Verification items for the finished model (mm, model axes). Face numbers are marked on the shaded views. A direction names the side the tool comes from. Round coordinates to 2 decimals unless told otherwise and drop trailing zeros. Order: outer loops, then holes, each group sorted by start corner. A loop starts at its lowest first (then second) coordinate and runs counter-clockwise, first axis right, second up. Notation, with made-up numbers: M 39.25,13.25 L 71.25,13.25 A23 cw 71.25,37.25 Z; hole C -13.5,-25 d3. An arc over 180 degrees is marked long. Use CSV: the item, a comma, the result in double quotes. Start each with the question number.
Q1. Sectioned sample at C-C (x = 8.25). Enter the section's corners in (y, z).
Q2. Gauge pin test, flat end, axial feed: pin 1 Ø3 at (x, z) = (2, 6.5) entering from -Y. Record the tip position at first contact, or that the pin passes through.
Q3. Set-up check for the marked faces 1 and 2: record each of +Z, -Z, +X, -X, +Y, -Y from which the full face is reachable in a straight line by a thin tool's end or side.
Q4. Scan lines: line 1 (Y direction, x = 8.5, z = 5); line 2 (X direction, y = 15, z = 8); line 3 (Y direction, x = 10, z = 4). Record each from-to range of solid material in increasing order.
Q5. Sectioned sample at A-A (y = 10). Enter the section's corners in (x, z), and give its area (3 significant figures).
Q6. Sectioned sample at B-B (z = 2). Enter the section's corners in (x, y).
Q7. Mould release check, pull along X, two halves, no side actions. Record for the marked faces 3, 4, 5 and 6: +X half, -X half, draft (parallel to the pull), parting line (faces both ways), or undercut.
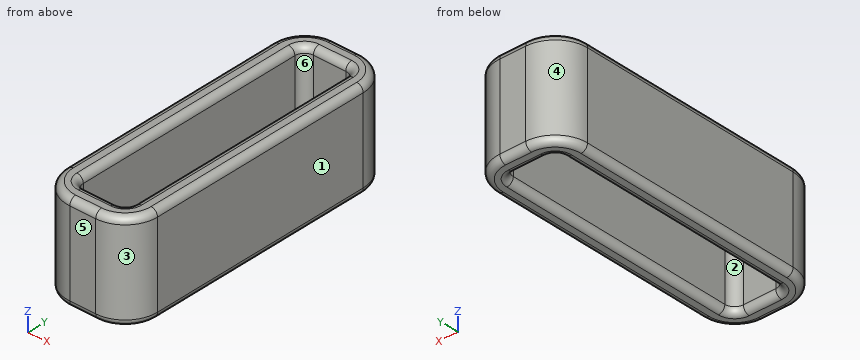
```python
from build123d import *

# Parameters (mm, degrees)
PAD_DEPTH = 15
FILLET_R  = 1


with BuildPart() as part:
    # Sketch → Pad (new body)
    with BuildSketch(Plane.XY):
        with BuildLine():
            Line((5, 0), (9, 0))
            ThreePointArc((9, 0), (12.535534, 1.464466), (14, 5))
            Line((14, 5), (14, 40))
            ThreePointArc((14, 40), (12.535534, 43.535534), (9, 45))
            Line((9, 45), (5, 45))
            ThreePointArc((5, 45), (1.464466, 43.535534), (0, 40))
            Line((0, 40), (0, 5))
            ThreePointArc((0, 5), (1.464466, 1.464466), (5, 0))
        make_face()
        with BuildLine():
            Line((4.5, 3), (9.5, 3))
            ThreePointArc((9.5, 3), (10.56066, 3.43934), (11, 4.5))
            Line((11, 4.5), (11, 40.5))
            ThreePointArc((11, 40.5), (10.56066, 41.56066), (9.5, 42))
            Line((9.5, 42), (4.5, 42))
            ThreePointArc((4.5, 42), (3.43934, 41.56066), (3, 40.5))
            Line((3, 40.5), (3, 4.5))
            ThreePointArc((3, 4.5), (3.43934, 3.43934), (4.5, 3))
        make_face(mode=Mode.SUBTRACT)
    extrude(amount=PAD_DEPTH)

    # Fillet
    fillet_edges = [part.edges().sort_by_distance(p)[0] for p in [
        (11, 22.5, 15),
        (14, 22.5, 15),
        (14, 22.5, 0),
        (11, 22.5, 0),
    ]]
    fillet(fillet_edges, radius=FILLET_R)


solid = part.part
```
Verdict:
1,outline,"M 0,1 A1 ccw 1,0 L 2,0 A1 ccw 3,1 L 3,14 A1 ccw 2,15 L 1,15 A1 ccw 0,14 Z; M 42,1 A1 ccw 43,0 L 44,0 A1 ccw 45,1 L 45,14 A1 ccw 44,15 L 43,15 A1 ccw 42,14 Z"
2,pin 1,"stops at y = 0.23"
3,face 1,"+Z, -Z, +X, +Y, -Y"
3,face 2,"+Z, -Z"
4,line 1,"y = 0 to 3, 42 to 45"
4,line 2,"x = 0 to 3, 11 to 14"
4,line 3,"y = 0.1 to 3.09, 41.91 to 44.9"
5,outline,"M 0,1 A1 ccw 1,0 L 2,0 A1 ccw 3,1 L 3,14 A1 ccw 2,15 L 1,15 A1 ccw 0,14 Z; M 11,1 A1 ccw 12,0 L 13,0 A1 ccw 14,1 L 14,14 A1 ccw 13,15 L 12,15 A1 ccw 11,14 Z"
5,area,"88.3 mm²"
6,outline,"M 0,5 A5 ccw 5,0 L 9,0 A5 ccw 14,5 L 14,40 A5 ccw 9,45 L 5,45 A5 ccw 0,40 Z; hole M 3,4.5 A1.5 ccw 4.5,3 L 9.5,3 A1.5 ccw 11,4.5 L 11,40.5 A1.5 ccw 9.5,42 L 4.5,42 A1.5 ccw 3,40.5 Z"
7,face 3,"+X half"
7,face 4,"-X half"
7,face 5,"draft"
7,face 6,"undercut"
